Can you work these out from the model? Positions are in its coordinate system, mm. Round coordinates to 2 decimals unless told otherwise and drop trailing zeros. Write each loop counter-clockwise with the first axis right and the second up, starting at its lowest first coordinate (ties: lowest second). Pieces come first, ordered by that corner, then holes. Notation, with made-up numbers: M 23.5,-28.75 L 67.5,-28.75 A19 cw 67.5,-13.75 Z; hole C -16,-20 d3. An arc over 180 degrees is marked long. Answer as a JSON object with one key per item and string values. Group by question number.
1) Suppose I cut it at C-C, the plane x = 0. Write out the boundary of the cut face in (y, z) (3 decimals), and give its area (3 significant figures).
2) Suppose I cut it at A-A, the plane z = 0. Write out the boundary of the cut face in (x, y) (3 decimals).
3) Please list where these lines run through material, in increasing order: L1, parallel to Z at x = 0, y = -2.3 (3 decimals); L2, parallel to X at y = -1, z = -0.5; L3, parallel to X at y = -0.05, z = 3. Write a range as [from, to].
4) If we mould it in two halves opening along X, with no side actions, what happens to faces 1 (the cylindrical face through (-24.95, -1.61, 24.92)), 2 (the cylindrical face through (7.559, -1.565, -5.796)), 3 (the flat face through (0, -2, -25.4)), 4 (the flat face through (25.4, -2, 0))? For each: +X half, -X half, draft (parallel to the pull), parting line (faces both ways), or undercut.
from build123d import *

# Parameters (mm, degrees)
F0_W     = 50.8
F0_H     = 50.8
F1_DEPTH = 3.175
F2_R     = 1.5875
F3_R     = 9.525
F4_DEPTH = 3.176


with BuildPart() as f1:
    # F0 (on Front) → F1 (new body)
    with BuildSketch(Plane.XZ):
        Rectangle(F0_W, F0_H)
    extrude(amount=F1_DEPTH)

    # F2
    f2_edges = [f1.edges().sort_by_distance(p)[0] for p in [
        (25.4, -1.5875, 25.4),
        (-25.4, -1.5875, 25.4),
        (-25.4, -1.5875, -25.4),
        (25.4, -1.5875, -25.4),
    ]]
    fillet(f2_edges, radius=F2_R)

    # F3 (on face) → F4 (cut, through all)
    with BuildSketch(Plane(origin=(0, 0, 0), x_dir=(-1, 0, 0), z_dir=(0, 1, 0))):
        Circle(F3_R)
    extrude(amount=-F4_DEPTH, mode=Mode.SUBTRACT)


solid = f1.part
Results:
{
 "1": {"outline": "M -3.175,-25.4 L 0,-25.4 L 0,-9.525 L -3.175,-9.525 Z; M -3.175,9.525 L 0,9.525 L 0,25.4 L -3.175,25.4 Z", "area": "101 mm^2"},
 "2": {"outline": "M -25.4,-3.175 L -9.525,-3.175 L -9.525,0 L -25.4,0 Z; M 9.525,-3.175 L 25.4,-3.175 L 25.4,0 L 9.525,0 Z"},
 "3": {"L1": "[-25.4, -9.525], [9.525, 25.4]", "L2": "[-25.4, -9.51], [9.51, 25.4]", "L3": "[-25.4, -9.04], [9.04, 25.4]"},
 "4": {"face 1": "-X half", "face 2": "undercut", "face 3": "draft", "face 4": "+X half"}
}
